Geometry check sheet. Reference: the model listing, model coordinates, mm. A direction names the side the tool comes from. Coordinates: 2 decimals unless noted, no trailing zeros. Order: outer loops, then holes, each group sorted by start corner. A loop starts at its lowest first (then second) coordinate and runs counter-clockwise, first axis right, second up. Notation, with made-up numbers: M 60.5,34 L 67.5,34 A16 cw 67.5,56 Z; hole C -3,68 d10. An arc over 180 degrees is marked long. One line per item, written item: value. Start each with the question number.
1) Sectioned sample at B-B, the plane y = -10.5. Enter the section's corners in (x, z).
2) Sectioned sample at C-C, the plane z = 0.65. Enter the section's corners in (x, y), then the cut area to 3 significant figures.
3) Go/stop test with a flat-tipped pin: P1, Ø1.5, axis at x = -0.5, y = -11, coming from the +Z side. Record where the tip stops, or that it passes through.
4) Access from +Z, -Z, +X, -X, +Y, -Y to the whole of each face (thin tool, end or side, straight path). Record for faces 1 (the flat face through (-2, 4, 0.3)), 2 (the flat face through (0, -1, 0)).
5) Thickness scan on L1, parallel to Z at x = 0.5, y = -10.5; L2, parallel to X at y = -1.75, z = 0.7; L3, parallel to Z at x = 0.25, y = -3.5. Record the ranges inside material, lowest first. Write a range as from..to.
6) Sectioned sample at A-A, the plane x = 0. Enter the section's corners in (y, z), then the cut area to 3 significant figures.
7) Sectioned sample at D-D, the plane y = -5. Enter the section's corners in (x, z) (3 decimals), then the cut area to 3 significant figures.
```python
from build123d import *

# Parameters (mm, degrees)
EXTRUDE_1_DEPTH  = 0.3
SKETCH_2_R       = 2.5
EXTRUDE_2_DEPTH  = 1
CHAMFER_1_SIZE   = 1.732050808
CHAMFER_1_SIZE_2 = 1


with BuildPart() as part:
    # 草图1 → 凸台-拉伸1 (new body)
    with BuildSketch(Plane.XY):
        with BuildLine():
            Line((-8, 0), (-8, 8))
            Line((-8, 8), (8, 8))
            Line((8, 8), (8, 0))
            ThreePointArc((8, 0), (6.164414003, -5.099019514), (1.5, -7.858116823))
            Line((1.5, -7.858116823), (1.5, -15.858116823))
            Line((1.5, -15.858116823), (-1.5, -15.858116823))
            Line((-1.5, -15.858116823), (-1.5, -7.858116823))
            ThreePointArc((-1.5, -7.858116823), (-6.164414003, -5.099019514), (-8, 0))
        make_face()
    extrude(amount=EXTRUDE_1_DEPTH)

    # 草图2 → 凸台-拉伸2 (add)
    with BuildSketch(Plane.XY.offset(0.3)):
        Circle(SKETCH_2_R)
    extrude(amount=EXTRUDE_2_DEPTH)

    # 倒角1
    # the kernel refuses this chamfer: 1.732050808, 1 mm, written as the material it adds along each edge
    with BuildSketch(Plane(origin=(0, 0, 0.3), x_dir=(1, 0, 0), z_dir=(0, -1, 0))) as chamfer_1_piece_1_section:
        Polygon((2.5 + CHAMFER_1_SIZE, 0), (2.5, CHAMFER_1_SIZE_2), (2.5, 0), align=None)
    chamfer_1_piece_1 = revolve(axis=Axis((0, 0, 0.3), (0, 0, 1)), mode=Mode.PRIVATE)
    chamfer_1_piece_1 = split(chamfer_1_piece_1, bisect_by=Plane(origin=(-3.382683679, 0, 1.3), z_dir=(0, 0, -1)), keep=Keep.TOP, mode=Mode.PRIVATE)
    add(chamfer_1_piece_1)


solid = part.part
```
Final values:
1. outline: M -1.5,0 L 1.5,0 L 1.5,0.3 L -1.5,0.3 Z
2. outline: C 0,0 d7.25
2. area: 41.3 mm^2
3. P1: stops at z = 0.3
4. face 1: +Z
4. face 2: -Z, +X, -X, +Y, -Y
5. L1: z = 0..0.3
5. L2: x = -3.08..3.08
5. L3: z = 0..0.72
6. outline: M -15.86,0 L 8,0 L 8,0.3 L 4.23,0.3 L 2.5,1.3 L -2.5,1.3 L -4.23,0.3 L -15.86,0.3 Z
6. area: 13.9 mm^2
7. outline: M -6.245,0 L 6.245,0 L 6.245,0.3 L -6.245,0.3 Z
7. area: 3.75 mm^2
